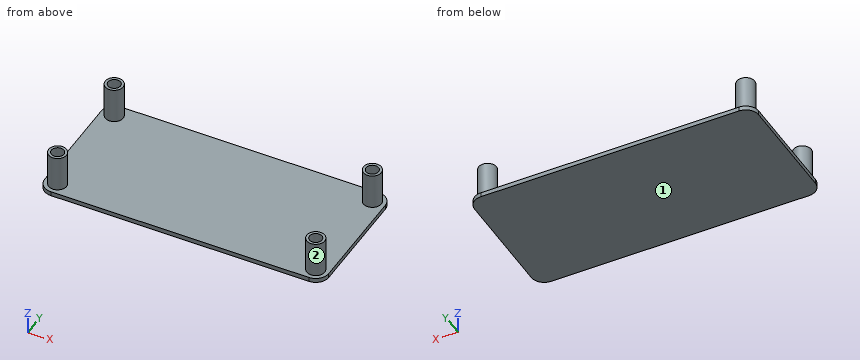
```python
from build123d import *

# Parameters (mm, degrees)
EXTRUDE_1_DEPTH = 1
SKETCH_3_R      = 2
SKETCH_3_R_2    = 1.4
EXTRUDE_3_DEPTH = 9


with BuildPart() as part:
    # 草图1 → 凸台-拉伸1 (new body)
    with BuildSketch(Plane.XY):
        with BuildLine():
            Line((0, -2.9), (57.7, -2.9))
            ThreePointArc((57.7, -2.9), (59.750609665, -2.050609665), (60.6, 0))
            Line((60.6, 0), (60.6, 24.1))
            ThreePointArc((60.6, 24.1), (59.750609665, 26.150609665), (57.7, 27))
            Line((57.7, 27), (0, 27))
            ThreePointArc((0, 27), (-2.050609665, 26.150609665), (-2.9, 24.1))
            Line((-2.9, 24.1), (-2.9, 0))
            ThreePointArc((-2.9, 0), (-2.050609665, -2.050609665), (0, -2.9))
        make_face()
    extrude(amount=EXTRUDE_1_DEPTH)

    # 草图3 → 凸台-拉伸3 (add)
    with BuildSketch(Plane.XY):
        Circle(SKETCH_3_R)
        Circle(SKETCH_3_R_2, mode=Mode.SUBTRACT)
        with Locations((0, 24.1)):
            Circle(SKETCH_3_R)
        with Locations((0, 24.1)):
            Circle(SKETCH_3_R_2, mode=Mode.SUBTRACT)
        with Locations((57.7, 0)):
            Circle(SKETCH_3_R)
        with Locations((57.7, 0)):
            Circle(SKETCH_3_R_2, mode=Mode.SUBTRACT)
        with Locations((57.7, 24.1)):
            Circle(SKETCH_3_R)
        with Locations((57.7, 24.1)):
            Circle(SKETCH_3_R_2, mode=Mode.SUBTRACT)
    extrude(amount=EXTRUDE_3_DEPTH)


solid = part.part
```
Can you work these out from the model? Positions are in its coordinate system, mm. Face numbers are marked on the shaded views. Give positions to 0.01 mm unless a question says otherwise; leave off trailing zeros. Order: outer loops, then holes, each group sorted by start corner. A loop starts at its lowest first (then second) coordinate and runs counter-clockwise, first axis right, second up. Notation, with made-up numbers: M 25.25,-17 L 79.25,-17 A29 ccw 79.25,19 Z; hole C 13,1 d9. An arc over 180 degrees is marked long. One line per item, written item: value.
1) I want a section at B-B, the plane x = 35. List the corners of the cut face in (y, z) for me.
Answer sheet:
outline: M -2.9,0 L 27,0 L 27,1 L -2.9,1 Z
2) I want a section at A-A, the plane z = 4.5. List the corners of the cut face in (x, y) for me, plus the area to 3 significant figures.
Answer sheet:
outline: C 0,0 d4; C 0,24.1 d4; C 57.7,0 d4; C 57.7,24.1 d4; hole C 0,0 d2.8; hole C 0,24.1 d2.8; hole C 57.7,0 d2.8; hole C 57.7,24.1 d2.8
area: 25.6 mm^2
3) I want a section at C-C, the plane y = 19.5. List the corners of the cut face in (x, z) for me, plus the area to 3 significant figures.
Answer sheet:
outline: M -2.9,0 L 60.6,0 L 60.6,1 L -2.9,1 Z
area: 63.5 mm^2
4) Please list where these lines run through material, in increasing order: line 1 along X through (y, z) = (24.1, 4.75); line 2 along Y through (x, z) = (0, 5.75); line 3 along Z through (x, y) = (17, 25).
Answer sheet:
line 1: x = -2 to -1.4, 1.4 to 2, 55.7 to 56.3, 59.1 to 59.7
line 2: y = -2 to -1.4, 1.4 to 2, 22.1 to 22.7, 25.5 to 26.1
line 3: z = 0 to 1
5) We'd pull the mould along Y, two halves only. Please class the marked faces 1 and 2: released by +Y, released by -Y, zero draft, split by the parting line, or undercut.
Answer sheet:
face 1: zero draft
face 2: undercut
6) For P1, Ø2, axis at y = 0.5, z = 3.5, coming from the -X side; P2, Ø2, axis at x = 0, y = 0.5, coming from the +Z side; P3, Ø2.5, axis at x = 0, y = 0, coming from the +Z side, each with a flat end and sliding along its axis, tell me the tip position at first contact or that it passes through.
Answer sheet:
P1: stops at x = -2
P2: stops at z = 9
P3: stops at z = 1
